```python
from build123d import *

# Parameters (mm, degrees)
SKETCH1_R           = 4.75
BOSS_EXTRUDE1_DEPTH = 14
BOSS_EXTRUDE2_DEPTH = 3
BOSS_EXTRUDE3_DEPTH = 3
SKETCH4_R           = 5
BOSS_EXTRUDE4_DEPTH = 15
SKETCH5_R           = 5
BOSS_EXTRUDE5_DEPTH = 106


with BuildPart() as part:
    # Sketch1 → Boss-Extrude1 (new body)
    with BuildSketch(Plane(origin=(0, 72.5, 0), x_dir=(1, 0, 0), z_dir=(0, 1, 0))):
        with Locations(Location((0, -26, 0), (0, 0, 270))):
            Circle(SKETCH1_R)
    extrude(amount=BOSS_EXTRUDE1_DEPTH)

    # Sketch2 → Boss-Extrude2 (add)
    with BuildSketch(Plane(origin=(0, 73.5, 0), x_dir=(1, 0, 0), z_dir=(0, 1, 0))):
        Polygon((8.082903769, -26), (4.041451884, -19), (-4.041451884, -19), (-8.082903769, -26), (-4.041451884, -33), (4.041451884, -33), align=None)
    extrude(amount=BOSS_EXTRUDE2_DEPTH)

    # Sketch3 → Boss-Extrude3 (add)
    with BuildSketch(Plane(origin=(0, 82.5, 0), x_dir=(1, 0, 0), z_dir=(0, 1, 0))):
        Polygon((8.082903769, -26), (4.041451884, -19), (-4.041451884, -19), (-8.082903769, -26), (-4.041451884, -33), (4.041451884, -33), align=None)
    extrude(amount=BOSS_EXTRUDE3_DEPTH)

    # Sketch4 → Boss-Extrude4 (add)
    with BuildSketch(Plane(origin=(0, 86.5, 0), x_dir=(1, 0, 0), z_dir=(0, 1, 0))):
        with Locations(Location((0, -26, 0), (0, 0, 270))):
            Circle(SKETCH4_R)
    extrude(amount=BOSS_EXTRUDE4_DEPTH)

    # Sketch5 → Boss-Extrude5 (add)
    with BuildSketch(Plane(origin=(0, 101.5, 0), x_dir=(1, 0, 0), z_dir=(0, 1, 0))):
        with Locations(Location((0, -26, 0), (0, 0, 270))):
            Circle(SKETCH5_R)
    extrude(amount=BOSS_EXTRUDE5_DEPTH)


solid = part.part
```
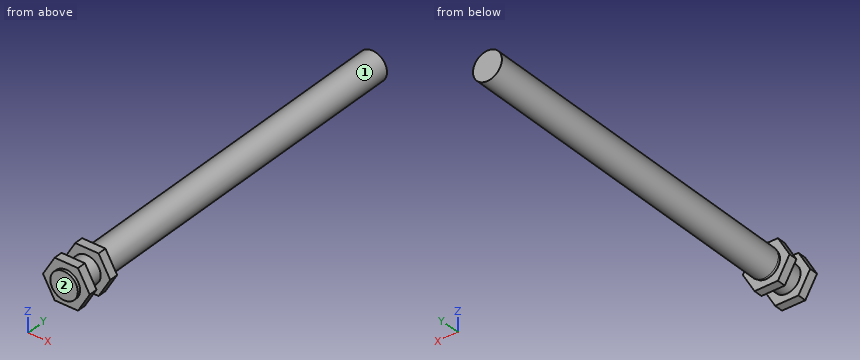
CAD build for the part. Positions are in the model's coordinates, mm. Face numbers are marked on the shaded views. A direction names the side the tool comes from. Round coordinates to 2 decimals unless told otherwise and drop trailing zeros. Order: outer loops, then holes, each group sorted by start corner. A loop starts at its lowest first (then second) coordinate and runs counter-clockwise, first axis right, second up. Notation, with made-up numbers: (9, 28) - (68, 28) arc R24 ccw to (68, 38) - close; hole circle Ø1 at (19, -4.75). An arc over 180 degrees is marked (long way). Use CSV: the item, a comma, the result in double quotes. Start each with the question number.
1) Tool access for the marked faces 1 and 2: list every direction of +Z, -Z, +X, -X, +Y, -Y with a clear straight run to the whole face (end or side of a thin tool).
2) Wall check: L1, parallel to Y at x = -5.5, z = 30; L2, parallel to X at y = 130, z = 25.75; L3, parallel to Z at x = 0.5, y = 142. Give the ranges that are in metal, low to high. Write a range as [from, to].
3) Saw through at C-C (y = 181.5). List the corners of the cut face in (x, z).
4) Saw through at A-A (x = 0). List the corners of the cut face in (y, z).
5) Saw through at B-B (z = 28.25). List the corners of the cut face in (x, y).
6) Pin check, flat tips, straight feed: pin 1 Ø1 at (x, z) = (4, 30) entering from -Y; pin 2 Ø1.5 at (y, z) = (86.5, 27.5) entering from +X; pin 3 Ø6 at (x, y) = (-5.5, 117) entering from +Z. Stop position of each tip, or through.
Values follow:
1,face 1,"+Y"
1,face 2,"+Z, -Z, +X, -X, -Y"
2,L1,"y = [73.5, 76.5], [82.5, 85.5]"
2,L2,"x = [-4.99, 4.99]"
2,L3,"z = [21.03, 30.97]"
3,outline,"circle Ø10 at (0, 26)"
4,outline,"(72.5, 21.25) - (73.5, 21.25) - (73.5, 19) - (76.5, 19) - (76.5, 21.25) - (82.5, 21.25) - (82.5, 19) - (85.5, 19) - (85.5, 21.25) - (86.5, 21.25) - (86.5, 21) - (207.5, 21) - (207.5, 31) - (86.5, 31) - (86.5, 30.75) - (85.5, 30.75) - (85.5, 33) - (82.5, 33) - (82.5, 30.75) - (76.5, 30.75) - (76.5, 33) - (73.5, 33) - (73.5, 30.75) - (72.5, 30.75) - close"
5,outline,"(-6.78, 73.5) - (-4.18, 73.5) - (-4.18, 72.5) - (4.18, 72.5) - (4.18, 73.5) - (6.78, 73.5) - (6.78, 76.5) - (4.18, 76.5) - (4.18, 82.5) - (6.78, 82.5) - (6.78, 85.5) - (4.18, 85.5) - (4.18, 86.5) - (4.47, 86.5) - (4.47, 207.5) - (-4.47, 207.5) - (-4.47, 86.5) - (-4.18, 86.5) - (-4.18, 85.5) - (-6.78, 85.5) - (-6.78, 82.5) - (-4.18, 82.5) - (-4.18, 76.5) - (-6.78, 76.5) - close"
6,pin 1,"stops at y = 73.5"
6,pin 2,"stops at x = 4.94"
6,pin 3,"stops at z = 30.33"
